Can you work these out from the model? Positions are in its coordinate system, mm. Give positions to 0.01 mm unless a question says otherwise; leave off trailing zeros. Order: outer loops, then holes, each group sorted by start corner. A loop starts at its lowest first (then second) coordinate and runs counter-clockwise, first axis right, second up. Notation, with made-up numbers: M 19,54 L 26,54 A28 cw 26,78 Z; hole C -33.75,-21 d8. An arc over 180 degrees is marked long. Answer as a JSON object with one key per item and string values.
```python
from build123d import *

# Parameters (mm, degrees)
SKETCH_1_W      = 92.2
SKETCH_1_H      = 42.5
EXTRUDE_1_DEPTH = 22.6
FILLET_1_R      = 2
SKETCH_6_R      = 1.5
SKETCH_6_W      = 15
SKETCH_6_H      = 6
EXTRUDE_5_DEPTH = 3


with BuildPart() as part:
    # 草图1 → 凸台-拉伸1 (new body)
    with BuildSketch(Plane(origin=(0, 0, 0), x_dir=(1, 0, 0), z_dir=(0, 1, 0))):
        Rectangle(SKETCH_1_W, SKETCH_1_H)
    extrude(amount=EXTRUDE_1_DEPTH)

    # 圆角1
    fillet_1_edges = [part.edges().sort_by_distance(p)[0] for p in [
        (0, 22.6, 21.25),
        (0, 0, 21.25),
        (0, 0, -21.25),
        (0, 22.6, -21.25),
    ]]
    fillet(fillet_1_edges, radius=FILLET_1_R)

    # 草图6 → 凸台-拉伸5 (add)
    with BuildSketch(Plane.ZY.offset(46.1)):
        with Locations(Location((-16, 4, 0), (0, 0, 180))):
            Circle(SKETCH_6_R)
        with Locations((7.5, 14.6)):
            Rectangle(SKETCH_6_W, SKETCH_6_H)
    extrude(amount=EXTRUDE_5_DEPTH)


solid = part.part
```
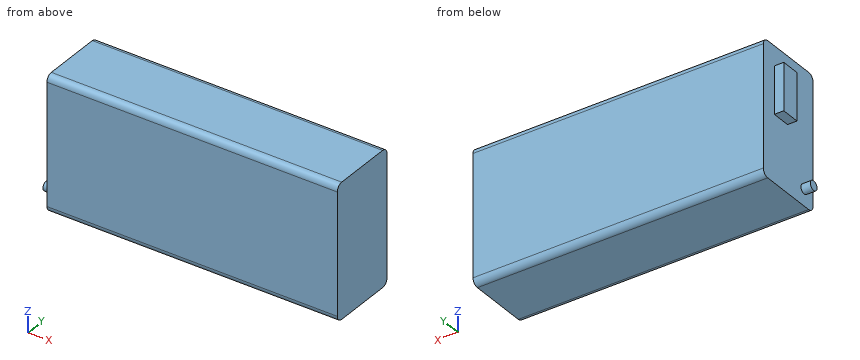
1) I need wall thicknesses on L1, parallel to Z at x = -6, y = 20.75; L2, parallel to X at y = 11.5, z = 18.5; L3, parallel to Y at x = -10.5, z = 19.5. Which ranges of each line are inside material? Lowest first, please.
Results found:
{"L1": "z = -21.24 to 21.24", "L2": "x = -46.1 to 46.1", "L3": "y = 0.02 to 22.58"}
2) I'm going to push flat-ended pins straight in: pin 1 Ø1.5 at (y, z) = (12.5, -5) entering from -X; pin 2 Ø0.9 at (x, y) = (-47.5, 14.5) entering from +Z. Where does each tip first touch, or does it pass through?
Results found:
{"pin 1": "stops at x = -46.1", "pin 2": "stops at z = 15"}
3) I want a section at B-B on y = 4. Write out the boundary of the cut face in (x, z).
Results found:
{"outline": "M -49.1,-17.5 L -46.1,-17.5 L -46.1,-21.25 L 46.1,-21.25 L 46.1,21.25 L -46.1,21.25 L -46.1,-14.5 L -49.1,-14.5 Z"}
4) I want a section at D-D on y = 7.75. Write out the boundary of the cut face in (x, z), and give its area (3 significant figures).
Results found:
{"outline": "M -46.1,-21.25 L 46.1,-21.25 L 46.1,21.25 L -46.1,21.25 Z", "area": "3,920 mm²"}
5) I want a section at A-A on z = 1. Write out the boundary of the cut face in (x, y), and give its area (3 significant figures).
Results found:
{"outline": "M -49.1,11.6 L -46.1,11.6 L -46.1,0 L 46.1,0 L 46.1,22.6 L -46.1,22.6 L -46.1,17.6 L -49.1,17.6 Z", "area": "2,100 mm²"}
6) I want a section at C-C on z = -7.5. Write out the boundary of the cut face in (x, y).
Results found:
{"outline": "M -46.1,0 L 46.1,0 L 46.1,22.6 L -46.1,22.6 Z"}
